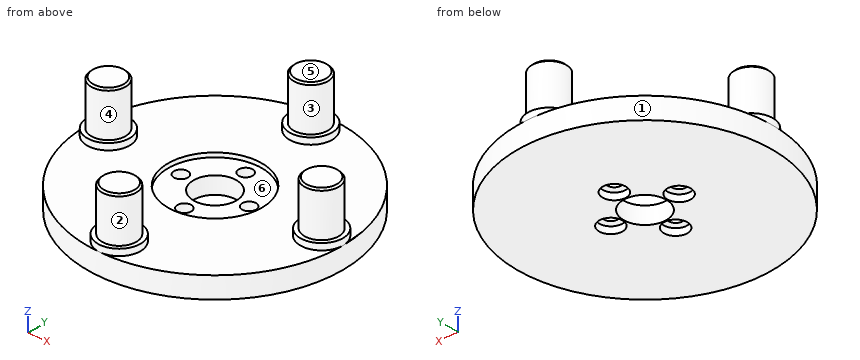
Solid Edge part; units mm, degrees
sketch "Sketch1" plane through (0, 0, 0) normal (0, 0, 1) x (1, 0, 0)
  circle A0 centre (8, 0) radius 1.625
  circle A1 centre (-8, 0) radius 1.625
  circle A2 centre (0, 0) radius 30
  circle A3 centre (0, 8) radius 1.625
  circle A4 centre (0, -8) radius 1.625
  circle A5 centre (0, 0) radius 5.05
extrude "Protrusion1" add sketch "Sketch1" along normal blind 5
sketch "Sketch2" plane through (0, 0, 5) normal (0, 0, 1) x (1, 0, 0)
  circle A0 centre (0, 0) radius 5.05
  circle A1 centre (0, 8) radius 1.625
  circle A2 centre (8, 0) radius 1.625
  circle A3 centre (0, -8) radius 1.625
  circle A4 centre (-8, 0) radius 1.625
  circle A5 centre (0, 0) radius 11.05
extrude "ExtrudedCutout_1" cut sketch "Sketch2" against normal blind 1
sketch "Sketch3" plane through (0, 0, 5) normal (0, 0, 1) x (1, 0, 0)
  circle A0 centre (-25, 0) radius 4.025
  circle A1 centre (0, 25) radius 4.025
  circle A2 centre (25, 0) radius 4.025
  circle A3 centre (0, -25) radius 4.025
extrude "ExtrudedProtrusion_2" add sketch "Sketch3" along normal blind 12
chamfer "Chamfer_2" distance 0.4 angle 45 4 edges at (-29.025, 0, 17) (-4.025, 25, 17) (-4.025, -25, 17) (20.975, 0, 17)
sketch "Sketch4" plane through (0, 0, 5) normal (0, 0, 1) x (1, 0, 0)
  circle A0 centre (25, 0) radius 5
  circle A1 centre (25, 0) radius 4.025
  circle A2 centre (0, 25) radius 5
  circle A3 centre (0, 25) radius 4.025
  circle A4 centre (0, -25) radius 5
  circle A5 centre (0, -25) radius 4.025
  circle A6 centre (-25, 0) radius 5
  circle A7 centre (-25, 0) radius 4.025
extrude "ExtrudedProtrusion_3" add sketch "Sketch4" along normal blind 1.5
sketch "Sketch5" plane through (0, 0, 0) normal (0, 0, 1) x (1, 0, 0)
  circle A0 centre (0, -8) radius 2.75
  circle A1 centre (0, -8) radius 1.625
  circle A2 centre (8, 0) radius 2.75
  circle A3 centre (8, 0) radius 1.625
  circle A4 centre (-8, 0) radius 2.75
  circle A5 centre (-8, 0) radius 1.625
  circle A6 centre (0, 8) radius 2.75
  circle A7 centre (0, 8) radius 1.625
extrude "Cutout1" cut sketch "Sketch5" along normal blind 2.0974
chamfer "Chamfer_3" distance 0.5 distance2 1.5 4 edges at (-10.75, 0, 2.0974) (-2.75, -8, 2.0974) (5.25, 0, 2.0974) (-2.75, 8, 2.0974) measured on face at (1.5218, -5.7095, 1.7269) measured on face at (-6.4782, 2.2905, 1.7269) measured on face at (9.5218, 2.2905, 1.7269) measured on face at (1.5218, 10.2905, 1.7269)
Can you work these out from the model? Positions are in its coordinate system, mm. Face numbers are marked on the shaded views. A direction names the side the tool comes from. Coordinates: 2 decimals unless noted, no trailing zeros. Order: outer loops, then holes, each group sorted by start corner. A loop starts at its lowest first (then second) coordinate and runs counter-clockwise, first axis right, second up.
1. If we section it at C-C (x = 25): Please give me the cut outline in (y, z) (3 decimals), then the cut area to 3 significant figures.
2. I need wall thicknesses on line 1 (Y direction, x = 0, z = 2.75) (3 decimals); line 2 (Y direction, x = 0, z = 0.3); line 3 (Z direction, x = 18.5, y = -21.5). Which ranges of each line are inside material? Lowest first, please.
3. Thinking about a two-plate mould opening in X: for the marked faces 3, 4, 5 and 6, which applies, +X half, -X half, draft (parallel to the pull), parting line (faces both ways), or undercut?
4. For the marked faces 1 and 2, which set-ups out of +Z, -Z, +X, -X, +Y, -Y let a thin tool reach every point of the face, with its end or its side?
5. I'm going to push flat-ended pins straight in: pin 1 (6.5 mm diameter, centred on x = 0, y = 8, fed in from +Z); pin 2 (6 mm diameter, centred on x = -5.5, z = 10.5, fed in from -Y); pin 3 (10 mm diameter, centred on x = -21.5, z = 12.5, fed in from -Y) (3 decimals); pin 4 (1 mm diameter, centred on x = -19.5, z = 13.5, fed in from +Y). Where does each tip first touch, or does it pass through?
6. If we section it at D-D (y = 13): Please give me the cut outline in (x, z), then the cut area to 3 significant figures.
7. If we section it at B-B (z = 8.75): Please give me the cut outline in (x, y) (3 decimals), then the cut area to 3 significant figures.
Entries:
1. outline: (-16.583, 0) - (16.583, 0) - (16.583, 5) - (5, 5) - (5, 6.5) - (4.025, 6.5) - (4.025, 16.6) - (3.625, 17) - (-3.625, 17) - (-4.025, 16.6) - (-4.025, 6.5) - (-5, 6.5) - (-5, 5) - (-16.583, 5) - close
1. area: 265 mm2
2. line 1: y = -30 to -9.625, -6.375 to -5.05, 5.05 to 6.375, 9.625 to 30
2. line 2: y = -30 to -10.75, -5.25 to -5.05, 5.05 to 5.25, 10.75 to 30
2. line 3: z = 0 to 5
3. face 3: parting line
3. face 4: undercut
3. face 5: draft
3. face 6: undercut
4. face 1: +Z, -Z
4. face 2: +Z
5. pin 1: stops at z = 5
5. pin 2: stops at y = -28.15
5. pin 3: stops at y = -4.025
5. pin 4: passes through
6. outline: (-27.04, 0) - (27.04, 0) - (27.04, 5) - (-27.04, 5) - close
6. area: 270 mm2
7. outline: circle Ø8.05 at (-25, 0); circle Ø8.05 at (0, -25); circle Ø8.05 at (0, 25); circle Ø8.05 at (25, 0)
7. area: 204 mm2
